Input: part model. Units: mm. Frame: model coordinates. Face numbers are marked on the shaded views. A direction names the side the tool comes from. Coordinates: 2 decimals unless noted, no trailing zeros. Order: outer loops, then holes, each group sorted by start corner. A loop starts at its lowest first (then second) coordinate and runs counter-clockwise, first axis right, second up. Notation, with made-up numbers: (0.25, 29) -> (30.25, 29) arc R35 cw to (30.25, 67) -> close; hole circle Ø4 at (-31.75, 26.25). An arc over 180 degrees is marked (long way). Write each question's results on one line, items separated by ' | '.
```python
from build123d import *

# Parameters (mm, degrees)
BOSS_EXTRUDE1_DEPTH = 6.35
FILLET1_R           = 2.54
CUT_EXTRUDE1_REACH  = 16.027
SKETCH2_R           = 1.7859375
SKETCH4_W           = 6.35
SKETCH4_H           = 2.04
BOSS_EXTRUDE3_DEPTH = 3.55
SKETCH6_R           = 2.1
BOSS_EXTRUDE5_DEPTH = 2.5
FILLET3_R           = 2.54


with BuildPart() as part:
    # Sketch1 → Boss-Extrude1 (new body)
    with BuildSketch(Plane.XY):
        Polygon((0, 6.04), (5.5, 6.04), (5.5, 2.04), (11.85, 2.04), (11.85, 0), (3.55, 0), (3.55, 4), (0, 4), align=None)
    extrude(amount=BOSS_EXTRUDE1_DEPTH)

    # Fillet1
    fillet1_edges = [part.edges().sort_by_distance(p)[0] for p in [
        (5.5, 6.04, 3.175),
        (11.85, 1.02, 6.35),
        (11.85, 1.02, 0),
    ]]
    fillet(fillet1_edges, radius=FILLET1_R)

    # Sketch2 → Cut-Extrude1 (cut, up to next)
    with BuildSketch(Plane(origin=(0, 2.04, 0), x_dir=(1, 0, 0), z_dir=(0, 1, 0)), mode=Mode.PRIVATE) as cut_extrude1_sk1:
        with Locations(Location((8, -3.175, 0), (0, 0, 270))):
            Circle(SKETCH2_R)
    cut_extrude1_tool1 = extrude(cut_extrude1_sk1.sketch, amount=-CUT_EXTRUDE1_REACH, mode=Mode.PRIVATE) & part.part
    add(cut_extrude1_tool1.solids().sort_by_distance((8, 2.04, 3.175))[0], mode=Mode.SUBTRACT)

    # Sketch4 → Boss-Extrude3 (add)
    with BuildSketch(Plane.ZY):
        with Locations((3.175, 5.02)):
            Rectangle(SKETCH4_W, SKETCH4_H)
    extrude(amount=BOSS_EXTRUDE3_DEPTH)

    # Sketch6 → Boss-Extrude5 (add)
    with BuildSketch(Plane.XZ.offset(-4)):
        with Locations(Location((0, 3.175, 0), (0, 0, 180))):
            Circle(SKETCH6_R)
    extrude(amount=BOSS_EXTRUDE5_DEPTH)

    # Fillet3
    fillet3_edges = [part.edges().sort_by_distance(p)[0] for p in [
        (-3.55, 5.02, 6.35),
        (-3.55, 5.02, 0),
    ]]
    fillet(fillet3_edges, radius=FILLET3_R)


solid = part.part
```
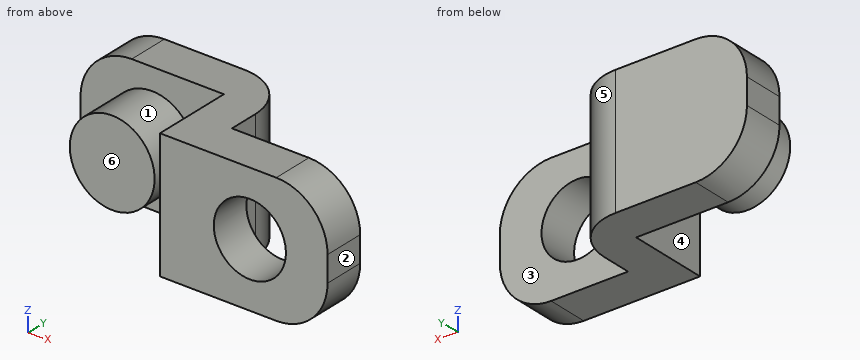
(1) Pin query (flat end, axial travel): P1, Ø2, axis at y = 2, z = 2.5, coming from the -X side; P2, Ø2, axis at y = 4, z = 4.5, coming from the +X side; P3, Ø2, axis at x = 0.5, z = 3, coming from the -Y side. Return the tip coordinate at first contact, or that it passes through.
Return value:
P1: x = -2.1 | P2: x = 5.5 | P3: y = 1.5
(2) Cut plane A-A, the plane x = 8. Return loops of the section in (y, z), plus the area to 3 significant figures.
Return value:
outline: (0, 0) -> (2.04, 0) -> (2.04, 1.39) -> (0, 1.39) -> close; (0, 4.96) -> (2.04, 4.96) -> (2.04, 6.35) -> (0, 6.35) -> close | area: 5.67 mm2
(3) Reachability of the marked faces 1, 2 and 3 from +Z, -Z, +X, -X, +Y, -Y: full face, straight path, thin tool, end or side. Return the list, or none.
Return value:
face 1: -Y | face 2: +Z, -Z, +X, +Y, -Y | face 3: +Z, -Z, +X, +Y
(4) Line query: line 1 along Y through (x, z) = (-2, 4.25); line 2 along Y through (x, z) = (-1, 2.25); line 3 along X through (y, z) = (1, 3.25). Output: solid intervals per line, ascending. Write a range as from..to.
Return value:
line 1: 4..6.04 | line 2: 1.5..6.04 | line 3: 3.55..6.22, 9.78..11.85
(5) Cut plane C-C, the plane z = 2.25. Return loops of the section in (x, y), plus the area to 3 significant figures.
Return value:
outline: (-3.53, 4) -> (-1.89, 4) -> (-1.89, 1.5) -> (1.89, 1.5) -> (1.89, 4) -> (3.55, 4) -> (3.55, 0) -> (6.47, 0) -> (6.47, 2.04) -> (5.5, 2.04) -> (5.5, 3.5) arc R2.54 ccw to (2.96, 6.04) -> (-3.53, 6.04) -> close; (9.53, 0) -> (11.83, 0) -> (11.83, 2.04) -> (9.53, 2.04) -> close | area: 41.0 mm2
(6) Mould query, pull axis X, two halves, no side actions, for the marked faces 4, 5 and 6. Classes: +X half, -X half, draft (parallel to the pull), parting line (faces both ways), or undercut.
Return value:
face 4: undercut | face 5: +X half | face 6: draft
(7) Cut plane D-D, the plane x = 0. Return loops of the section in (y, z) (3 decimals).
Return value:
outline: (1.5, 1.075) -> (4, 1.075) -> (4, 0) -> (6.04, 0) -> (6.04, 6.35) -> (4, 6.35) -> (4, 5.275) -> (1.5, 5.275) -> close
(8) Cut plane B-B, the plane y = 1. Return loops of the section in (x, z) (3 decimals), plus the area to 3 significant figures.
Return value:
outline: (3.55, 0) -> (9.31, 0) arc R2.54 ccw to (11.85, 2.54) -> (11.85, 3.81) arc R2.54 ccw to (9.31, 6.35) -> (3.55, 6.35) -> close; hole circle Ø3.572 at (8, 3.175) | area: 39.9 mm2
